from build123d import *

# Parameters (mm, degrees)
SKETCH1_R                 = 15
SKETCH1_R_2               = 1.5875
SKETCH1_R_3               = 4
BOSS_EXTRUDE2_DEPTH       = 10
F_6_32_TAPPED_HOLE1_D     = 2.7051
F_6_32_TAPPED_HOLE1_DEPTH = 14.999
F_6_32_TAPPED_HOLE1_TIP   = 0.81269403


with BuildPart() as part:
    # Sketch1 → Boss-Extrude2 (new body)
    with BuildSketch(Plane.XY):
        Circle(SKETCH1_R)
        with Locations((0, 10)):
            Circle(SKETCH1_R_2, mode=Mode.SUBTRACT)
        Circle(SKETCH1_R_3, mode=Mode.SUBTRACT)
        with Locations((0, -10)):
            Circle(SKETCH1_R_2, mode=Mode.SUBTRACT)
    extrude(amount=BOSS_EXTRUDE2_DEPTH)

    # #6-32 Tapped Hole1
    with Locations(Plane(origin=(15, 0, 4.999999906), x_dir=(0, 1, 0), z_dir=(1, 0, 0))):
        with Locations((0, 0)):
            Hole(F_6_32_TAPPED_HOLE1_D / 2, depth=F_6_32_TAPPED_HOLE1_DEPTH)
            with Locations((0, 0, -(F_6_32_TAPPED_HOLE1_DEPTH + F_6_32_TAPPED_HOLE1_TIP / 2))):  # 118° drill point
                Cone(0, F_6_32_TAPPED_HOLE1_D / 2, F_6_32_TAPPED_HOLE1_TIP, mode=Mode.SUBTRACT)


solid = part.part
Geometry check sheet. Reference: the model listing, model coordinates, mm. A direction names the side the tool comes from. Coordinates: 2 decimals unless noted, no trailing zeros. Order: outer loops, then holes, each group sorted by start corner. A loop starts at its lowest first (then second) coordinate and runs counter-clockwise, first axis right, second up. Notation, with made-up numbers: (31, 23) - (61, 23) arc R20 cw to (61, 43) - close; hole circle Ø1 at (30.5, -30). An arc over 180 degrees is marked (long way). One line per item, written item: value.
(1) Sectioned sample at D-D (z = 4). Enter the section's corners in (x, y) (1 decimal).
Data:
outline: (3.9, -0.9) arc R4 cw (long way) to (3.9, 0.9) - (15, 0.9) arc R15 ccw (long way) to (15, -0.9) - close; hole circle Ø3.2 at (0, -10); hole circle Ø3.2 at (0, 10)
(2) Sectioned sample at A-A (y = 0). Enter the section's corners in (x, z).
Data:
outline: (-15, 0) - (-4, 0) - (-4, 10) - (-15, 10) - close; (4, 0) - (15, 0) - (15, 3.65) - (4, 3.65) - close; (4, 6.35) - (15, 6.35) - (15, 10) - (4, 10) - close
(3) Release check for a two-part mould opening along X. For faces 1 (the face through (3, -3, 0)), 2 (the face through (-14.985, 0.66, 4.93)), 3 (the face through (0.73, 8.59, 4.93)) record: +X half, -X half, draft (parallel to the pull), parting line (faces both ways), or undercut.
Data:
face 1: draft
face 2: parting line
face 3: undercut
(4) Thickness scan on probe 1 along Y at (x, z) = (3, 2); probe 2 along Y at (x, z) = (11, 4); probe 3 along X at (y, z) = (13, 0.75). Record the ranges inside material, lowest first. Write a range as from..to.
Data:
probe 1: y = -14.7..-2.65, 2.65..14.7
probe 2: y = -10.2..-0.91, 0.91..10.2
probe 3: x = -7.48..7.48
(5) Sectioned sample at B-B (x = -1). Enter the section's corners in (y, z), and give its area (3 significant figures).
Data:
outline: (-14.97, 0) - (-11.23, 0) - (-11.23, 10) - (-14.97, 10) - close; (-8.77, 0) - (-3.87, 0) - (-3.87, 10) - (-8.77, 10) - close; (3.87, 0) - (8.77, 0) - (8.77, 10) - (3.87, 10) - close; (11.23, 0) - (14.97, 0) - (14.97, 10) - (11.23, 10) - close
area: 173 mm^2
(6) Sectioned sample at C-C (y = -9). Enter the section's corners in (x, z), and give its area (3 significant figures).
Data:
outline: (-12, 0) - (-1.23, 0) - (-1.23, 10) - (-12, 10) - close; (1.23, 0) - (12, 0) - (12, 10) - (1.23, 10) - close
area: 215 mm^2
(7) Depth check by flat-ended pin: pin 1 Ø3 at (y, z) = (-10.5, 4) entering from -X; pin 2 Ø2 at (x, z) = (-12, 8) entering from -Y; pin 3 Ø1.5 at (y, z) = (3, 7.5) entering from +X. Enter the tip coordinate at first touch or a pass-through.
Data:
pin 1: stops at x = -12
pin 2: stops at y = -10.2
pin 3: stops at x = 14.83
(8) Access from +Z, -Z, +X, -X, +Y, -Y to the whole of each face (thin tool, end or side, straight path). Record for faces 4 (the face through (9.3, 0.29, 3.68)), 5 (the face through (3, -3, 10)).
Data:
face 4: +X
face 5: +Z, +X, -X, +Y, -Y
